from build123d import *


with BuildPart() as part:
    # Sketch2 → Revolve2 (revolve)
    with BuildSketch(Plane.XY, mode=Mode.PRIVATE) as revolve2_sk:
        with BuildLine():
            Line((0, 0), (20, 0))
            ThreePointArc((20, 0), (20.382866953, 0.92432259), (21.307189542, 1.307189542))
            add(Edge.make_bspline(
                [(21.307189542, 1.307189542), (50.589297326, -3.648702918), (80, 5.283333405)],
                knots=[0, 0, 0, 1, 1, 1], degree=2))
            ThreePointArc((80, 5.283333405), (79.644135668, 4.296719594), (78.771253816, 3.715235711))
            Line((78.771253816, 3.715235711), (66.216017581, -0.934527379))
            add(Edge.make_bspline(
                [(16, -9.716666595), (31.973399001, -2.802481332), (50.081212283, -7.497100863), (66.216017581, -0.934527379)],
                knots=[0, 0, 0, 0, 1, 1, 1, 1], degree=3))
            Line((16, -9.716666595), (0, -9.716666595))
            Line((0, -9.716666595), (0, 0))
        make_face()
    revolve(revolve2_sk.sketch.rotate(Axis((0, 0, 0), (0, -1, 0)), 180), axis=Axis((0, 0, 0), (0, -1, 0)))


solid = part.part
Could you check a few things on this model? Use its own coordinates, in mm. Give positions to 0.01 mm unless a question says otherwise; leave off trailing zeros.
Item 1: If we mould it in two halves opening along Z, with no side actions, what happens to faces 1 (the face through (0, -9.717, 0)), 2 (the face through (-63.74, -0.71, -20.07)), 3 (the face through (0, 0, 0))? For each: pulls with the +Z half, pulls with the -Z half, needs draft (parallel to the pull), parting line crosses it, or undercut.
Item 2: I'm going to push flat-ended pins straight in: pin 1 (1 mm diameter, centred on x = 22, z = 26, fed in from -Y); pin 2 (6 mm diameter, centred on x = 31.5, z = 26.5, fed in from -Y); pin 3 (3 mm diameter, centred on y = 3, z = -60, fed in from +X). Where does each tip first touch, or does it pass through?
Item 3: I need wall thicknesses on line 1 (Y direction, x = 2.5, z = -35); line 2 (Y direction, x = 53, z = -13). Which ranges of each line are inside material? Lowest first, please.
Values:
1. face 1: needs draft
1. face 2: parting line crosses it
1. face 3: undercut
2. pin 1: stops at y = -5.73
2. pin 2: stops at y = -5.37
2. pin 3: stops at x = 53.27
3. line 1: y = -5.59 to -0.26
3. line 2: y = -3.99 to 0.15
